Design review of the part shown in the three views and the two pictorial views. Dimensions are in mm from the part's minimum x, y and z. Give positions to 0.01 mm unless a question says otherwise; leave off trailing zeros. Loops run counter-clockwise (first coordinate to the right, second up) from the corner with the lowest first, then second, coordinate; pieces in that order, holes last. Notation, with made-up numbers: (39, 22.5) - (49, 22.5) arc R22 ccw to (49, 30.5) - close; hole circle Ø9 at (21, 65). An arc over 180 degrees is marked (long way). Use CSV: the item, a comma, the result in double quotes. Start each with the question number.
1. Wall thickness on line 1 (Z direction, x = 9, y = 51.4); line 2 (X direction, y = 52, z = 25); line 3 (Z direction, x = 41, y = 36): over which ranges is each line inside the solid? List them lowest first.
2. Take a section at B-B on y = 13.5. Give the boundary of the cut face in (x, z).
3. Take a section at D-D on y = 8. Give the boundary of the cut face in (x, z).
4. Take a section at A-A on z = 18.5. Give the boundary of the cut face in (x, y).
5. For pin 1 (6 mm diameter, centred on x = 32, y = 30.5, fed in from -Z); pin 2 (4 mm diameter, centred on y = 21.5, z = 27.5, fed in from -X), all flat-tipped, find the tip position at first contact; note any pin that passes through.
6. Mouldability with a two-part tool opening along Z and no side actions: class the marked faces 1, 2, 3 and 4 as pulls with the +Z half, pulls with the -Z half, needs draft (parallel to the pull), parting line crosses it, or undercut.
7. Take a section at C-C on x = 9.5. State how many separate pieces and enclosed holes the cut face has, plus the area to 3 significant figures.
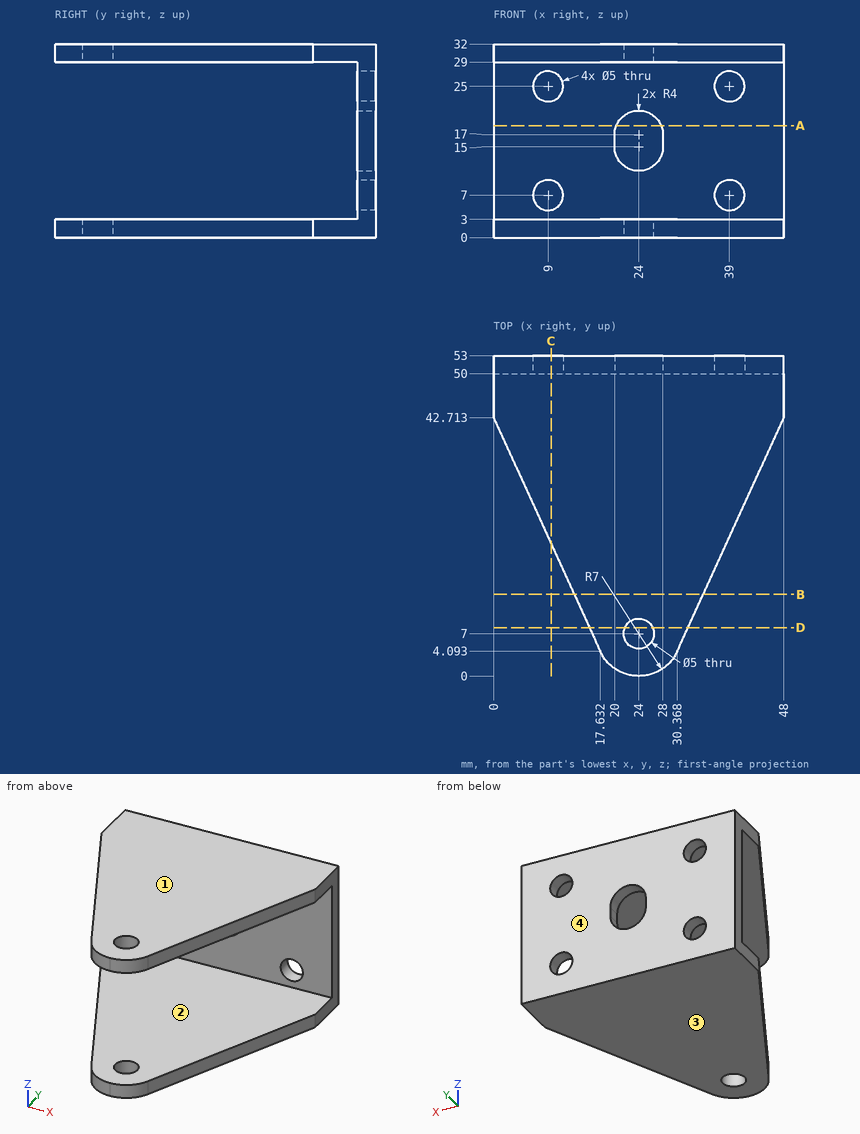
Check result:
1,line 1,"z = 0 to 4.5, 9.5 to 22.5, 27.5 to 32"
1,line 2,"x = 0 to 6.5, 11.5 to 36.5, 41.5 to 48"
1,line 3,"z = 0 to 3, 29 to 32"
2,outline,"(13.34, 0) - (34.66, 0) - (34.66, 3) - (13.34, 3) - close; (13.34, 29) - (34.66, 29) - (34.66, 32) - (13.34, 32) - close"
3,outline,"(15.85, 0) - (21.71, 0) - (21.71, 3) - (15.85, 3) - close; (15.85, 29) - (21.71, 29) - (21.71, 32) - (15.85, 32) - close; (26.29, 0) - (32.15, 0) - (32.15, 3) - (26.29, 3) - close; (26.29, 29) - (32.15, 29) - (32.15, 32) - (26.29, 32) - close"
4,outline,"(0, 50) - (20.29, 50) - (20.29, 53) - (0, 53) - close; (27.71, 50) - (48, 50) - (48, 53) - (27.71, 53) - close"
5,pin 1,"stops at z = 0"
5,pin 2,"stops at x = 9.08"
6,face 1,"pulls with the +Z half"
6,face 2,"undercut"
6,face 3,"pulls with the -Z half"
6,face 4,"needs draft"
7,separate pieces,"3"
7,enclosed holes,"0"
7,area,"235 mm²"
